```python
from build123d import *

# Parameters (mm, degrees)
F1_DEPTH = 30
F2_R     = 1
F5_DEPTH = 3
F6_DEPTH = 3


with BuildPart() as f1:
    # F0 (on Front) → F1 (new body)
    with BuildSketch(Plane.XZ):
        Polygon((18, -12.6854385647), (10, 11), (-10, 11), (-10, -11), (-8, -11), (-8, 9), (8.5645188749, 9), (16.1051649148, -13.3254385647), align=None)
    extrude(amount=F1_DEPTH)

    # F2
    f2_edges = [f1.edges().sort_by_distance(p)[0] for p in [
        (10, -15, 11),
        (-10, -15, 11),
        (-8, -15, 9),
        (8.564519, -15, 9),
    ]]
    fillet(f2_edges, radius=F2_R)

    # F3 (on face) → F5 (cut)
    with BuildSketch(Plane(origin=(12.3109097499, 0, 4.1581361363), x_dir=(0, 1, 0), z_dir=(0.9474175426, 0, 0.32))):
        with BuildLine():
            ThreePointArc((-12.5, -7.7784070316), (-16.767766953, -6.0106400786), (-15, -10.2784070316))
            ThreePointArc((-15, -10.2784070316), (-13.232233047, -9.5461739845), (-12.5, -7.7784070316))
        make_face()
    extrude(amount=-F5_DEPTH, mode=Mode.SUBTRACT)

    # F4 (on face) → F6 (cut)
    with BuildSketch(Plane(origin=(-10, 0, 0), x_dir=(0, -1, 0), z_dir=(-1, 0, 0))):
        with BuildLine():
            ThreePointArc((19, -1), (12.1715728753, 1.8284271247), (15, -5))
            ThreePointArc((15, -5), (17.8284271247, -3.8284271247), (19, -1))
        make_face()
    extrude(amount=-F6_DEPTH, mode=Mode.SUBTRACT)


solid = f1.part
```
For this review, take the finished solid that the model builds, in its own axes (mm). A direction names the side the tool comes from. Round coordinates to 2 decimals unless told otherwise and drop trailing zeros. Write each loop counter-clockwise with the first axis right and the second up, starting at its lowest first coordinate (ties: lowest second). Pieces come first, ordered by that corner, then holes. Notation, with made-up numbers: (-30.5, -10.75) - (-20.5, -10.75) arc R15 cw to (-20.5, -2.75) - close; hole circle Ø10 at (83.5, 20). An arc over 180 degrees is marked (long way). Put each result on its own line as item: value.
Q1. Wall thickness on probe 1 along Y at (x, z) = (-8.5, -1); probe 2 along Z at (x, y) = (-8.8, -15); probe 3 along Z at (x, y) = (3, -3.5): over which ranges is each line inside the solid? List them lowest first.
Solved:
probe 1: y = -30 to -19, -11 to 0
probe 2: z = -11 to -5, 3 to 11
probe 3: z = 9 to 11
Q2. Machinability: for faces 4 (the face through (-9.699, -15.21, 10.715)), 5 (the face through (0, -15, 9)), which of the approach directions +Z, -Z, +X, -X, +Y, -Y give a long, thin tool a straight path to every point of the face, cutting with its end or side? Answer none if there is none.
Solved:
face 4: +Z, -X, +Y, -Y
face 5: -Z, +Y, -Y
Q3. We need section B-B (z = 4). Give the boundary of the cut face in (x, y), and give its area (3 significant figures).
Solved:
outline: (-10, -30) - (-8, -30) - (-8, 0) - (-10, 0) - close; (10.25, -30) - (12.36, -30) - (12.36, 0) - (10.25, 0) - close
area: 123 mm2
Q4. Mouldability with a two-part tool opening along X and no side actions: class faces 1 (the face through (-9, -15, -11)), 2 (the face through (13.306, -14.79, 1.212)), 3 (the face through (11.586, -14.79, 0.054)) as released by +X, released by -X, zero draft, split by the parting line, or undercut.
Solved:
face 1: zero draft
face 2: released by +X
face 3: undercut
Q5. We need section D-D (x = -6). Give the boundary of the cut face in (y, z), and give its area (3 significant figures).
Solved:
outline: (-30, 9) - (0, 9) - (0, 11) - (-30, 11) - close
area: 60.0 mm2
Q6. Insertion check: pin 1 Ø4.5 at (x, y) = (2.5, -18.5) entering from -Z; pin 2 Ø5 at (x, y) = (12, -26.5) entering from +Z; pin 3 Ø1.6 at (x, y) = (-9.5, -8) entering from -Z. Each pin has a flat end and moves straight along its axis. Give the tip position at first contact, or say it passes through.
Solved:
pin 1: stops at z = 9
pin 2: stops at z = 10.98
pin 3: stops at z = -11
Q7. We need section A-A (y = -4). Give the boundary of the cut face in (x, z).
Solved:
outline: (-10, -11) - (-8, -11) - (-8, 8) arc R1 cw to (-7, 9) - (7.85, 9) arc R1 cw to (8.79, 8.32) - (16.11, -13.33) - (18, -12.69) - (10.23, 10.32) arc R1 ccw to (9.28, 11) - (-9, 11) arc R1 ccw to (-10, 10) - close
Q8. We need section C-C (y = -13.75). Give the boundary of the cut face in (x, z), and give its area (3 significant figures).
Solved:
outline: (-10, -11) - (-8, -11) - (-8, -4.8) - (-10, -4.8) - close; (-10, 2.8) - (-8, 2.8) - (-8, 8) arc R1 cw to (-7, 9) - (7.85, 9) arc R1 cw to (8.79, 8.32) - (12.21, -1.8) - (14.11, -1.16) - (10.23, 10.32) arc R1 ccw to (9.28, 11) - (-9, 11) arc R1 ccw to (-10, 10) - close; (13.6, -5.9) - (16.11, -13.33) - (18, -12.69) - (15.49, -5.26) - close
area: 103 mm2
